Model file for the job. Use its own axes, mm. Give positions to 0.01 mm unless a question says otherwise; leave off trailing zeros. Order: outer loops, then holes, each group sorted by start corner. A loop starts at its lowest first (then second) coordinate and runs counter-clockwise, first axis right, second up. Notation, with made-up numbers: (46.5, 79) -> (58.5, 79) arc R16 cw to (58.5, 86) -> close; hole circle Ø3 at (46, 9). An arc over 180 degrees is marked (long way). Use CSV: the item, a comma, the result in double quotes. Start each with the question number.
1. Drop flat-ended pins along their axis: pin 1 (6 mm diameter, centred on x = 44.245, y = -26, fed in from +Z) (3 decimals); pin 2 (1.5 mm diameter, centred on x = -3, z = -1, fed in from +Y). Give the stop position or say it passes through.
2. Wall check: line 1 (X direction, y = -26, z = -2.35) (3 decimals); line 2 (Y direction, x = 46.5, z = -0.5); line 3 (X direction, y = -50.5, z = -1.5) (3 decimals). Give the ranges that are in metal, low to high. Write a range as from..to.
3. Cut at C-C on y = -26. List the corners of the cut face in (x, z) (3 decimals), then the cut area to 3 significant figures.
4. Cut at D-D on z = -0.75. Give the number of separate pieces and of enclosed holes in the cut face, then the cut area to 3 significant figures.
5. Cut at A-A on x = 0. List the corners of the cut face in (y, z) (1 decimal), then the cut area to 3 significant figures.
6. Cut at B-B on y = -51. List the corners of the cut face in (x, z) (3 decimals), then the cut area to 3 significant figures.
```python
from build123d import *

# Parameters (mm, degrees)
SKETCH2_W                                       = 110.49
SKETCH2_H                                       = 6.35
BOSS_EXTRUDE1_DEPTH                             = 63.5
SKETCH3_R                                       = 14.43749998
CUT_EXTRUDE1_DEPTH                              = 85.407242136
CHAMFER1_SIZE                                   = 6.35
FILLET2_R                                       = 0.762
CSK_FOR_M5_FLAT_HEAD_MACHINE_SCREW1_D           = 5.3
CSK_FOR_M5_FLAT_HEAD_MACHINE_SCREW1_CSINK_D     = 10.4
CSK_FOR_M5_FLAT_HEAD_MACHINE_SCREW1_CSINK_ANGLE = 90


with BuildPart() as part:
    # Sketch2 → Boss-Extrude1 (new body)
    with BuildSketch(Plane(origin=(0, 0, 0), x_dir=(1, 0, 0), z_dir=(0, 1, 0))):
        Rectangle(SKETCH2_W, SKETCH2_H)
    extrude(amount=-BOSS_EXTRUDE1_DEPTH)

    # Sketch3 → Cut-Extrude1 (cut, through all)
    with BuildSketch(Plane.XY.offset(3.175)):
        with Locations((0, -28.8150046)):
            Circle(SKETCH3_R)
    extrude(amount=-CUT_EXTRUDE1_DEPTH, mode=Mode.SUBTRACT)

    # Chamfer1
    chamfer1_edges = [part.edges().sort_by_distance(p)[0] for p in [
        (55.245, 0, 0),
        (-55.245, 0, 0),
    ]]
    chamfer(chamfer1_edges, length=CHAMFER1_SIZE)

    # Fillet2
    fillet2_edges = [part.edges().sort_by_distance(p)[0] for p in [
        (55.245, -63.5, 0),
        (0, -63.5, -3.175),
        (0, 0, 3.175),
        (0, 0, -3.175),
        (48.895, 0, 0),
        (-48.895, 0, 0),
        (52.07, -3.175, 3.175),
        (-52.07, -3.175, 3.175),
        (-55.245, -6.35, 0),
        (52.07, -3.175, -3.175),
        (-52.07, -3.175, -3.175),
        (55.245, -6.35, 0),
        (-55.245, -63.5, 0),
        (-55.245, -34.925, -3.175),
        (55.245, -34.925, -3.175),
        (55.245, -34.925, 3.175),
        (-55.245, -34.925, 3.175),
        (0, -63.5, 3.175),
    ]]
    fillet(fillet2_edges, radius=FILLET2_R)

    # CSK for M5 Flat Head Machine Screw1 (through all)
    with Locations(Plane.XY.offset(3.175)):
        with Locations((-44.245, -26), (-44.245, -51), (44.245, -51), (44.245, -26)):
            CounterSinkHole(CSK_FOR_M5_FLAT_HEAD_MACHINE_SCREW1_D / 2, CSK_FOR_M5_FLAT_HEAD_MACHINE_SCREW1_CSINK_D / 2, counter_sink_angle=CSK_FOR_M5_FLAT_HEAD_MACHINE_SCREW1_CSINK_ANGLE)


solid = part.part
```
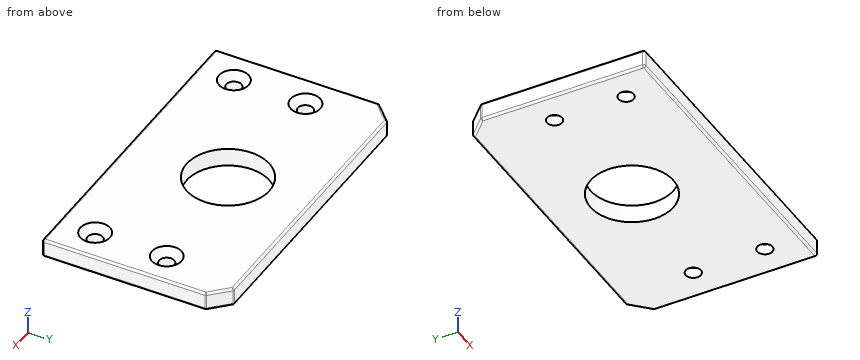
Verdict:
1,pin 1,"z = 0.975"
1,pin 2,"y = 0"
2,line 1,"-55.245..-46.895, -41.595..-14.16, 14.16..41.595, 46.895..55.245"
2,line 2,"-63.5..-52.39, -49.61..-27.39, -24.61..0"
2,line 3,"-55.245..-46.847, -41.643..41.643, 46.847..55.245"
3,outline,"(-55.245, -2.413) arc R0.762 ccw to (-54.483, -3.175) -> (-46.895, -3.175) -> (-46.895, 0.625) -> (-49.445, 3.175) -> (-54.483, 3.175) arc R0.762 ccw to (-55.245, 2.413) -> close; (-41.595, -3.175) -> (-14.16, -3.175) -> (-14.16, 3.175) -> (-39.045, 3.175) -> (-41.595, 0.625) -> close; (14.16, -3.175) -> (41.595, -3.175) -> (41.595, 0.625) -> (39.045, 3.175) -> (14.16, 3.175) -> close; (46.895, -3.175) -> (54.483, -3.175) arc R0.762 ccw to (55.245, -2.413) -> (55.245, 2.413) arc R0.762 ccw to (54.483, 3.175) -> (49.445, 3.175) -> (46.895, 0.625) -> close"
3,area,"441 mm^2"
4,separate pieces,"1"
4,enclosed holes,"5"
4,area,"6,230 mm^2"
5,outline,"(-63.5, -2.4) arc R0.8 ccw to (-62.7, -3.2) -> (-43.3, -3.2) -> (-43.3, 3.2) -> (-62.7, 3.2) arc R0.8 ccw to (-63.5, 2.4) -> close; (-14.4, -3.2) -> (-0.8, -3.2) arc R0.8 ccw to (0, -2.4) -> (0, 2.4) arc R0.8 ccw to (-0.8, 3.2) -> (-14.4, 3.2) -> close"
5,area,"219 mm^2"
6,outline,"(-55.245, -2.413) arc R0.762 ccw to (-54.483, -3.175) -> (-46.895, -3.175) -> (-46.895, 0.625) -> (-49.445, 3.175) -> (-54.483, 3.175) arc R0.762 ccw to (-55.245, 2.413) -> close; (-41.595, -3.175) -> (41.595, -3.175) -> (41.595, 0.625) -> (39.045, 3.175) -> (-39.045, 3.175) -> (-41.595, 0.625) -> close; (46.895, -3.175) -> (54.483, -3.175) arc R0.762 ccw to (55.245, -2.413) -> (55.245, 2.413) arc R0.762 ccw to (54.483, 3.175) -> (49.445, 3.175) -> (46.895, 0.625) -> close"
6,area,"621 mm^2"
